Autodesk Fusion 360 part; units mm, degrees
sketch "Sketch1" plane through (0, 0, 0) normal (0, 0, 1) x (1, 0, 0)
  circle A0 centre (0, 0) radius 40
  line L0 (39.8478, 3.4862) -> (278.222, 24.3413)
  line L1 (0, 0) -> (300, 0) construction
  line L2 (39.8478, -3.4862) -> (278.222, -24.3413)
  arc A1 (299.9627, -4.7329) -> (299.9627, 4.7329) centre (0, 0) ccw
  arc A2 (299.9627, 4.7329) -> (278.222, 24.3413) centre (279.9652, 4.4174) ccw
  arc A3 (278.222, -24.3413) -> (299.9627, -4.7329) centre (279.9652, -4.4174) ccw
  line L3 (25.7115, 30.6418) -> (179.5208, 213.9446)
  line L4 (30.6418, 25.7115) -> (213.9446, 179.5208)
  arc A4 (213.9446, 179.5208) -> (215.4523, 208.759) centre (201.0888, 194.8417) ccw
  arc A5 (215.4523, 208.759) -> (208.759, 215.4523) centre (0, 0) ccw
  arc A6 (208.759, 215.4523) -> (179.5208, 213.9446) centre (194.8417, 201.0888) ccw
  line L5 (-3.4862, 39.8478) -> (-24.3413, 278.222)
  line L6 (3.4862, 39.8478) -> (24.3413, 278.222)
  arc A7 (24.3413, 278.222) -> (4.7329, 299.9627) centre (4.4174, 279.9652) ccw
  arc A8 (4.7329, 299.9627) -> (-4.7329, 299.9627) centre (0, 0) ccw
  arc A9 (-4.7329, 299.9627) -> (-24.3413, 278.222) centre (-4.4174, 279.9652) ccw
  line L7 (-30.6418, 25.7115) -> (-213.9446, 179.5208)
  line L8 (-25.7115, 30.6418) -> (-179.5208, 213.9446)
  arc A10 (-179.5208, 213.9446) -> (-208.759, 215.4523) centre (-194.8417, 201.0888) ccw
  arc A11 (-208.759, 215.4523) -> (-215.4523, 208.759) centre (0, 0) ccw
  arc A12 (-215.4523, 208.759) -> (-213.9446, 179.5208) centre (-201.0888, 194.8417) ccw
  line L9 (-39.8478, -3.4862) -> (-278.222, -24.3413)
  line L10 (-39.8478, 3.4862) -> (-278.222, 24.3413)
  arc A13 (-278.222, 24.3413) -> (-299.9627, 4.7329) centre (-279.9652, 4.4174) ccw
  arc A14 (-299.9627, 4.7329) -> (-299.9627, -4.7329) centre (0, 0) ccw
  arc A15 (-299.9627, -4.7329) -> (-278.222, -24.3413) centre (-279.9652, -4.4174) ccw
  line L11 (-25.7115, -30.6418) -> (-179.5208, -213.9446)
  line L12 (-30.6418, -25.7115) -> (-213.9446, -179.5208)
  arc A16 (-213.9446, -179.5208) -> (-215.4523, -208.759) centre (-201.0888, -194.8417) ccw
  arc A17 (-215.4523, -208.759) -> (-208.759, -215.4523) centre (0, 0) ccw
  arc A18 (-208.759, -215.4523) -> (-179.5208, -213.9446) centre (-194.8417, -201.0888) ccw
  line L13 (3.4862, -39.8478) -> (24.3413, -278.222)
  line L14 (-3.4862, -39.8478) -> (-24.3413, -278.222)
  arc A19 (-24.3413, -278.222) -> (-4.7329, -299.9627) centre (-4.4174, -279.9652) ccw
  arc A20 (-4.7329, -299.9627) -> (4.7329, -299.9627) centre (0, 0) ccw
  arc A21 (4.7329, -299.9627) -> (24.3413, -278.222) centre (4.4174, -279.9652) ccw
  line L15 (30.6418, -25.7115) -> (213.9446, -179.5208)
  line L16 (25.7115, -30.6418) -> (179.5208, -213.9446)
  arc A22 (179.5208, -213.9446) -> (208.759, -215.4523) centre (194.8417, -201.0888) ccw
  arc A23 (208.759, -215.4523) -> (215.4523, -208.759) centre (0, 0) ccw
  arc A24 (215.4523, -208.759) -> (213.9446, -179.5208) centre (201.0888, -194.8417) ccw
  point P0 (298.8584, 26.1467)
  dimension "d1" = 80
  dimension "d3" = 5
  dimension "d4" = 300
  dimension "d5" = 20
  dimension "d6" = 20
  dimension "d8" = 360
extrude "Extrude1" add sketch "Sketch1" along normal blind 50 contours A0 L0 L2 A1 A2 A3 | A0 L3 L4 A4 A5 A6 | A0 L15 L16 A22 A23 A24 | A0 L5 L6 A7 A8 A9 | A0 L13 L14 A19 A20 A21 | A0 L7 L8 A10 A11 A12 | A0 L11 L12 A16 A17 A18 | A0 L9 L10 A13 A14 A15 makes body 1 at (-10.4379, 119.3059, 16.6667) makes body 2 at (10.4379, -119.3059, 16.6667) makes body 3 at (-76.9813, -91.7427, 16.6667) makes body 4 at (91.7427, 76.9813, 16.6667) makes body 5 at (-91.7427, 76.9813, 16.6667) makes body 6 at (76.9813, -91.7427, 16.6667) makes body 7 at (-119.3059, -10.4379, 16.6667) makes body 8 at (119.3059, 10.4379, 16.6667)
extrude "Extrude2" add sketch "Sketch1" along normal blind 80 contours A0 bodies 1 2 3 4 5 6 7 8
extrude "Extrude3" add 1 faces at (13.1844, -1.9872, 80) along direction (0, 0, 1) blind 300 on bodies 1 bodies 1
sketch "Sketch2" plane through (0, 0, 380) normal (0, 0, 1) x (-1, 0, 0)
  circle A0 centre (0, 0) radius 40
  circle A1 centre (0, 0) radius 25
  dimension "d15" = 50
extrude "Extrude4" cut sketch "Sketch2" against normal blind 280 contours A1 bodies 1
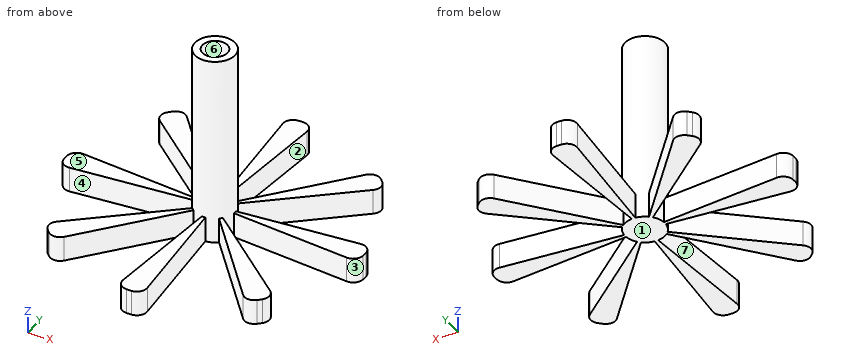
Geometry check sheet. Reference: the model listing, model coordinates, mm. Face numbers are marked on the shaded views. A direction names the side the tool comes from. Round coordinates to 2 decimals unless told otherwise and drop trailing zeros. Write each loop counter-clockwise with the first axis right and the second up, starting at its lowest first coordinate (ties: lowest second). Pieces come first, ordered by that corner, then holes. Notation, with made-up numbers: (13, 78.25) - (22, 78.25) arc R18 cw to (22, 107.25) - close; hole circle Ø4 at (-32.5, 18). An arc over 180 degrees is marked (long way). Write each question's results on one line, items separated by ' | '.
(1) Depth check by flat-ended pin: pin 1 Ø24.5 at (x, y) = (-190, 6) entering from +Z; pin 2 Ø4 at (y, z) = (4.5, 252.5) entering from -X; pin 3 Ø25 at (x, y) = (-10, -8.5) entering from +Z; pin 4 Ø1 at (x, z) = (15, 223) entering from -Y. Enter the tip coordinate at first touch or a pass-through.
Computed:
pin 1: stops at z = 50 | pin 2: stops at x = -39.92 | pin 3: stops at z = 380 | pin 4: stops at y = -37.28
(2) Thickness scan on probe 1 along Y at (x, z) = (0, 312); probe 2 along X at (y, z) = (198, 28.5). Record the ranges inside material, lowest first. Write a range as from..to.
Computed:
probe 1: y = -40..-25, 25..40 | probe 2: x = -220.84..-166.14, -17.32..17.32, 166.14..220.84
(3) Draft check along Y on the marked faces 1, 2, 3 and 4. Enter one of: pulls with the +Y half, pulls with the -Y half, needs draft (parallel to the pull), parting line crosses it, or undercut.
Computed:
face 1: needs draft | face 2: undercut | face 3: pulls with the -Y half | face 4: undercut
(4) Sectioned sample at A-A, the plane x = 88.5. Enter the section's corners in (y, z).
Computed:
outline: (-105.47, 0) - (-74.26, 0) - (-74.26, 50) - (-105.47, 50) - close; (-7.74, 0) - (7.74, 0) - (7.74, 50) - (-7.74, 50) - close; (74.26, 0) - (105.47, 0) - (105.47, 50) - (74.26, 50) - close
(5) Set-up check for the marked faces 5, 6 and 7: record each of +Z, -Z, +X, -X, +Y, -Y from which the full face is reachable in a straight line by a thin tool's end or side.
Computed:
face 5: +Z, -X, +Y, -Y | face 6: +Z | face 7: +Z, -Z
(6) Sectioned sample at C-C, the plane z = 163. Enter the section's corners in (x, y), plus the area to 3 significant figures.
Computed:
outline: circle Ø80 at (0, 0); hole circle Ø50 at (0, 0) | area: 3,060 mm^2
(7) Sectioned sample at B-B, the plane y = 72. Enter the section's corners in (x, z).
Computed:
outline: (-85.81, 0) - (-60.42, 0) - (-60.42, 50) - (-85.81, 50) - close; (-6.3, 0) - (6.3, 0) - (6.3, 50) - (-6.3, 50) - close; (60.42, 0) - (85.81, 0) - (85.81, 50) - (60.42, 50) - close
(8) Sectioned sample at D-D, the plane z = 79.5. Enter the section's corners in (x, y), plus the area to 3 significant figures.
Computed:
outline: circle Ø80 at (0, 0) | area: 5,030 mm^2
